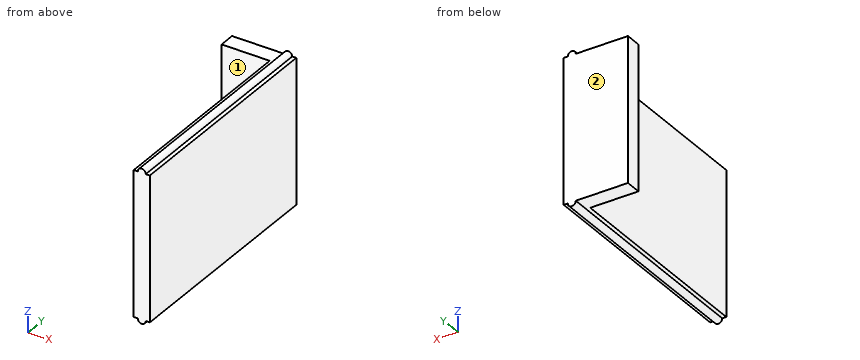
Autodesk Inventor part; units mm, degrees
ref_plane "YZ Plane" through (0, 0, 0) normal (1, 0, 0) x (0, 1, 0)
ref_plane "XZ Plane" through (0, 0, 0) normal (0, 1, 0) x (-1, 0, 0)
ref_plane "XY Plane" through (0, 0, 0) normal (0, 0, 1) x (1, 0, 0)
sketch "Sketch1" plane through (0, 0, 0) normal (0, 1, 0) x (-1, 0, 0)
  line L0 (0, 0) -> (25.4, 0)
  line L1 (25.4, 0) -> (25.4, -57.15)
  line L2 (25.4, -57.15) -> (0, -57.15)
  line L3 (0, -57.15) -> (0, 0)
  dimension "d0" = 25.4
  dimension "d1" = 57.15
extrude "Extrusion1" add sketch "Sketch1" along normal blind 88.9
sketch "Sketch2" plane through (0, 0, 0) normal (0, -1, 0) x (1, 0, 0)
  line L0 (0, 0) -> (-6.35, 0)
  line L1 (-25.4, 0) -> (0, 0)
  line L2 (-6.35, 0) -> (-6.35, -57.15)
  line L3 (0, -57.15) -> (-25.4, -57.15)
  line L4 (-6.35, 0) -> (-25.4, 0)
  line L5 (-25.4, -57.15) -> (-25.4, 0)
  line L6 (-25.4, -57.15) -> (-25.4, 0)
  line L7 (-25.4, -57.15) -> (-6.35, -57.15)
  dimension "d4" = 6.35
extrude "Extrusion2" cut sketch "Sketch2" against normal blind 82.55
sketch "Sketch3" plane through (0, 88.9, 0) normal (0, 1, 0) x (1, 0, 0)
  line L0 (0, 0) -> (0, 57.15)
  line L1 (0, 57.15) -> (-3.175, 57.15)
  line L2 (-6.35, 57.15) -> (0, 57.15)
  arc A0 (-1.5875, 57.15) -> (-4.7625, 57.15) centre (-3.175, 57.15) ccw
  line L3 (-4.7625, 57.15) -> (0, 57.15)
  arc A1 (-4.7625, 0) -> (-1.5875, 0) centre (-3.175, 0) ccw
  line L4 (-4.7625, 0) -> (-1.5875, 0)
  line L5 (0, 0) -> (-3.175, 0)
  dimension "d12" = 3.175
  dimension "d13" = 3.175
  dimension "d17" = 3.175
  dimension "d18" = 3.175
extrude "Extrusion3" add sketch "Sketch3" against normal blind 88.9
properties part number "arduinocase"
Work out the finished part from the listing and answer in its coordinate system (mm). Face numbers are marked on the shaded views. A direction names the side the tool comes from. Give positions to 0.01 mm unless a question says otherwise; leave off trailing zeros. Order: outer loops, then holes, each group sorted by start corner. A loop starts at its lowest first (then second) coordinate and runs counter-clockwise, first axis right, second up. Notation, with made-up numbers: (13, 43.5) -> (70, 43.5) arc R7 ccw to (70, 54.5) -> close; hole circle Ø6 at (50.25, 13.5). An arc over 180 degrees is marked (long way). Answer as CSV lines item,"result". Start each with the question number.
(1) Section C-C, the plane x = -16.5 is taken. Write down the section's boundary in (y, z), plus the area to 3 significant figures.
(2) Consider line 1 along Y through (x, z) = (-7.5, -16.5); line 2 along Z through (x, y) = (-0.75, 74); line 3 along X through (y, z) = (12, -6). Determine where each line is inside the solid, lowest interval first.
(3) Which of the six approach directions +Z, -Z, +X, -X, +Y, -Y give full straight-line access (tool end or side, diameter ignored) to the marked faces 1 and 2?
(4) Section B-B, the plane z = -11.5 is taken. Write down the section's boundary in (x, y), plus the area to 3 significant figures.
(5) Each of these flat-tipped pins is pushed along its axis until it touches: pin 1 Ø1.7 at (x, y) = (-1, 36.5) entering from +Z; pin 2 Ø9.5 at (x, z) = (-17, -40) entering from -Y; pin 3 Ø1 at (y, z) = (38, -51.5) entering from -X; pin 4 Ø4 at (x, z) = (-4.5, -15.5) entering from -Y. Where does it stop, or does it pass through?
Entries:
1,outline,"(82.55, -57.15) -> (88.9, -57.15) -> (88.9, 0) -> (82.55, 0) -> close"
1,area,"363 mm²"
2,line 1,"82.55 to 88.9"
2,line 2,"-57.15 to 0"
2,line 3,"-6.35 to 0"
3,face 1,"+Z, -Z, -X, -Y"
3,face 2,"+Z, -Z, +X, -X, +Y"
4,outline,"(-25.4, 82.55) -> (-6.35, 82.55) -> (-6.35, 0) -> (0, 0) -> (0, 88.9) -> (-25.4, 88.9) -> close"
4,area,"685 mm²"
5,pin 1,"z = 0.87"
5,pin 2,"y = 82.55"
5,pin 3,"x = -6.35"
5,pin 4,"y = 0"
